from build123d import *

# Parameters (mm, degrees)
F0_W     = 2000
F0_H     = 100
F1_DEPTH = 50
F3_R     = 5
F4_DEPTH = 25
F2_R     = 5
F5_DEPTH = 25
F5_TAPER = -3
F6_R     = 5
F7_DEPTH = 50


with BuildPart() as f1:
    # F0 (on Front) → F1 (new body)
    with BuildSketch(Plane.XZ):
        Rectangle(F0_W, F0_H)
    extrude(amount=F1_DEPTH)

    # F3 (on face) → F4 (cut)
    with BuildSketch(Plane(origin=(-1000, 0, 0), x_dir=(0, -1, 0), z_dir=(-1, 0, 0))):
        with Locations((25, 25)):
            Circle(F3_R)
        with Locations((25, -25)):
            Circle(F3_R)
    extrude(amount=-F4_DEPTH, mode=Mode.SUBTRACT)

    # F2 (on face) → F5 (cut)
    with BuildSketch(Plane.YZ.offset(1000)):
        with Locations((-25, -25)):
            Circle(F2_R)
        with Locations((-25, 25)):
            Circle(F2_R)
    extrude(amount=-F5_DEPTH, taper=F5_TAPER, mode=Mode.SUBTRACT)

    # F6 (on face) → F7 (cut)
    with BuildSketch(Plane.XZ.offset(50)):
        with Locations((-275, 40)):
            Circle(F6_R)
        with Locations((-275, -40)):
            Circle(F6_R)
        with Locations((275, 40)):
            Circle(F6_R)
        with Locations((275, -40)):
            Circle(F6_R)
    extrude(amount=-F7_DEPTH, mode=Mode.SUBTRACT)


solid = f1.part
Design review of the part built by this model. Coordinates are the model's own, in mm. Coordinates: 2 decimals unless noted, no trailing zeros. One line per item, written item: value.
1) To check wall thickness, follow probe 1 along Z at (x, y) = (-275, -15); probe 2 along Z at (x, y) = (-983.5, -25); probe 3 along X at (y, z) = (-41, 37). State the ranges of each line that lie inside material, in increasing order. Write a range as [from, to].
Output values:
probe 1: z = [-50, -45], [-35, 35], [45, 50]
probe 2: z = [-50, -30], [-20, 20], [30, 50]
probe 3: x = [-1000, -279], [-271, 271], [279, 1000]
2) Clearance check with flat-ended pins moving along their axes: P1, Ø3, axis at y = -26, z = -27, coming from the -X side; P2, Ø8, axis at y = -25, z = -25, coming from the +X side; P3, Ø6, axis at x = -275, z = -40, coming from the +Y side. State where each tip first meets the part, or that it passes through.
Output values:
P1: stops at x = -975
P2: stops at x = 975
P3: passes through
3) Draft analysis for pull direction Y (two halves, no side actions). For faces 1 (the face through (-14, -25, -50)), 2 (the face through (-14, 0, 1)), 3 (the face through (-14, -50, 1)), state which applies: +Y half, -Y half, draft (parallel to the pull), parting line (faces both ways), or undercut.
Output values:
face 1: draft
face 2: +Y half
face 3: -Y half
